The figure shows three views and two pictorial views of one solid part (mm, origin at its lowest corner). Answer the questions. A direction names the side the tool comes from. Round coordinates to 2 decimals unless told otherwise and drop trailing zeros. Loops run counter-clockwise (first coordinate to the right, second up) from the corner with the lowest first, then second, coordinate; pieces in that order, holes last. Notation, with made-up numbers: (54, -40) -> (109, -40) arc R30 cw to (109, -10) -> close; hole circle Ø11 at (40, 30.25). An arc over 180 degrees is marked (long way). Write item = value, one per line. Start each with the question number.
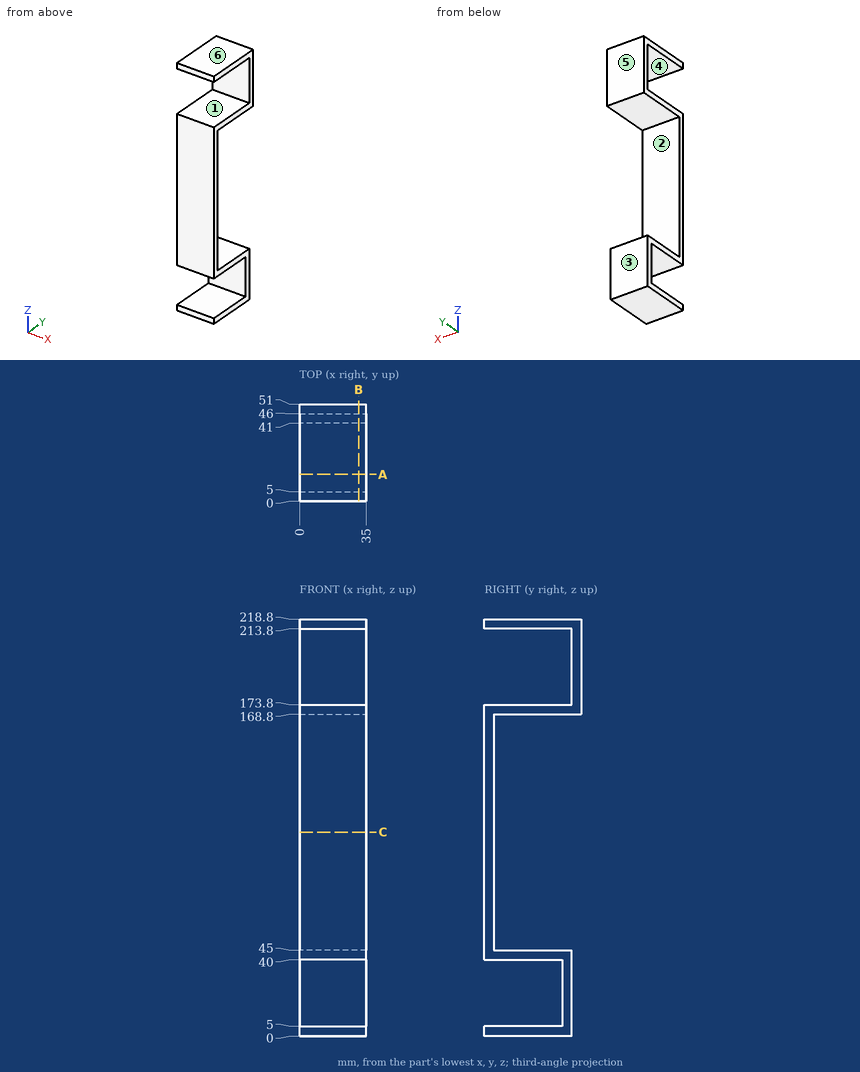
Item 1: Section A-A (y = 14) is taken. Determine the outline of the cut face in (x, z).
Item 2: Section B-B (x = 31) is taken. Determine the outline of the cut face in (y, z).
Item 3: A flat-ended cylindrical pin translates along its axis: pin 1 (3 mm diameter, centred on x = 23.5, z = 44.5, fed in from +Y). Find the tip coordinate at first contact, or state that the pin passes through.
Item 4: Section C-C (z = 107) is taken. Determine the outline of the cut face in (x, y).
Item 5: Find the intervals of material crossed by line 1 along Z through (x, y) = (26.5, 8.5); line 2 along Z through (x, y) = (12.5, 4.5); line 3 along Z through (x, y) = (32, 45.5), in increasing order. Write a range as [from, to].
Item 6: A tool of negligible diameter and unlimited length cuts with its end or side. For the marked faces 1, 2 and 3, from which of +Z, -Z, +X, -X, +Y, -Y can it reach the whole face along a straight path? Write none if from no direction.
Item 7: The mould has two halves that part along Z. Classify the marked faces 4, 5 and 6: pulls with the +Z half, pulls with the -Z half, needs draft (parallel to the pull), parting line crosses it, or undercut.
Worked answers:
q1.outline = (0, 0) -> (35, 0) -> (35, 5) -> (0, 5) -> close; (0, 40) -> (35, 40) -> (35, 45) -> (0, 45) -> close; (0, 168.8) -> (35, 168.8) -> (35, 173.8) -> (0, 173.8) -> close; (0, 213.8) -> (35, 213.8) -> (35, 218.8) -> (0, 218.8) -> close
q2.outline = (0, 0) -> (46, 0) -> (46, 45) -> (5, 45) -> (5, 168.8) -> (51, 168.8) -> (51, 218.8) -> (0, 218.8) -> (0, 213.8) -> (46, 213.8) -> (46, 173.8) -> (0, 173.8) -> (0, 40) -> (41, 40) -> (41, 5) -> (0, 5) -> close
q3.pin_1 = 46
q4.outline = (0, 0) -> (35, 0) -> (35, 5) -> (0, 5) -> close
q5.line_1 = [0, 5], [40, 45], [168.8, 173.8], [213.8, 218.8]
q5.line_2 = [0, 5], [40, 173.8], [213.8, 218.8]
q5.line_3 = [0, 45], [168.8, 173.8], [213.8, 218.8]
q6.face_1 = +X, -X, -Y
q6.face_2 = +X, -X, +Y
q6.face_3 = -Z, +X, -X, +Y
q7.face_4 = undercut
q7.face_5 = needs draft
q7.face_6 = pulls with the +Z half
